from build123d import *

# Parameters (mm, degrees)
SKETCH_1_W          = 40
SKETCH_1_H          = 40
EXTRUDE_1_DEPTH     = 9
SKETCH_2_W          = 5.7
SKETCH_2_H          = 40
EXTRUDE_2_DEPTH     = 40
CUT_EXTRUDE_START   = -40
CUT_EXTRUDE_2_DEPTH = 40
SKETCH_4_R          = 4
CUT_EXTRUDE_3_DEPTH = 67.340033162
SKETCH_5_R          = 8
CUT_EXTRUDE_4_DEPTH = 2
SKETCH_6_R          = 4
CUT_EXTRUDE_5_DEPTH = 49.989794856
SKETCH_7_W          = 8.2
SKETCH_7_H          = 1
EXTRUDE_3_DEPTH     = 2


# Read off the part's stored shape, not the designer's step: 切除-拉伸2
with BuildPart() as part:
    # 草图1 → 凸台-拉伸1 (new body)
    with BuildSketch(Plane.XY):
        Rectangle(SKETCH_1_W, SKETCH_1_H)
    extrude(amount=EXTRUDE_1_DEPTH)

    # 草图2 → 凸台-拉伸2 (add)
    with BuildSketch(Plane.XY.offset(9)):
        with Locations((-17.15, 0)):
            Rectangle(SKETCH_2_W, SKETCH_2_H)
        with Locations((17.15, 0)):
            Rectangle(SKETCH_2_W, SKETCH_2_H)
    extrude(amount=EXTRUDE_2_DEPTH)

    # 切除-拉伸2 outline → 切除-拉伸2 (cut)
    with BuildSketch(Plane.ZY.offset(20).offset(CUT_EXTRUDE_START)):
        with BuildLine():
            Line((49, 20), (29, 20))
            ThreePointArc((29, 20), (43.142135559, 14.142135688), (49, 1.83e-07))
            Line((49, 1.83e-07), (49, 20))
        make_face()
        with BuildLine():
            Line((49, -20), (49, 1.83e-07))
            ThreePointArc((49, 1.83e-07), (43.142135688, -14.142135559), (29, -20))
            Line((29, -20), (49, -20))
        make_face()
    extrude(amount=CUT_EXTRUDE_2_DEPTH, mode=Mode.SUBTRACT)

    # 草图4 → 切除-拉伸3 (cut, through all)
    with BuildSketch(Plane.ZY.offset(20)):
        with Locations((29, 0)):
            Circle(SKETCH_4_R)
    extrude(amount=-CUT_EXTRUDE_3_DEPTH, mode=Mode.SUBTRACT)

    # 草图5 → 切除-拉伸4 (cut)
    with BuildSketch(Plane.ZY.offset(20)):
        with Locations((29, 0)):
            Circle(SKETCH_5_R)
    extrude(amount=-CUT_EXTRUDE_4_DEPTH, mode=Mode.SUBTRACT)

    # 草图6 → 切除-拉伸5 (cut, through all)
    with BuildSketch(Plane.XY.offset(9)):
        Circle(SKETCH_6_R)
    extrude(amount=-CUT_EXTRUDE_5_DEPTH, mode=Mode.SUBTRACT)

    # 草图7 → 凸台-拉伸3 (add)
    with BuildSketch(Plane(origin=(0, 0, 0), x_dir=(-1, 0, 0), z_dir=(0, 0, -1))):
        with Locations((0, 19.5)):
            Rectangle(SKETCH_7_W, SKETCH_7_H)
        with Locations((0, -19.5)):
            Rectangle(SKETCH_7_W, SKETCH_7_H)
    extrude(amount=EXTRUDE_3_DEPTH)


solid = part.part
CAD build for the part. Positions are in the model's coordinates, mm. A direction names the side the tool comes from. Coordinates: 2 decimals unless noted, no trailing zeros. Write each loop counter-clockwise with the first axis right and the second up, starting at its lowest first coordinate (ties: lowest second). Pieces come first, ordered by that corner, then holes. Notation, with made-up numbers: M 41.25,34 L 52.25,34 A21 cw 52.25,67 Z; hole C 8,86.5 d6. An arc over 180 degrees is marked long. Answer as a JSON object with one key per item and string values. Group by question number.
1) Tool access for faces 1 (the face through (-20, 0, 19)), 2 (the face through (0, -19, -1)), 3 (the face through (-19, 0, 21)), 4 (the face through (-14.3, 0, 24)): list every direction of +Z, -Z, +X, -X, +Y, -Y with a clear straight run to the whole face (end or side of a thin tool).
2) Pin check, flat tips, straight feed: pin 1 Ø8 at (x, z) = (7, 39.5) entering from -Y; pin 2 Ø6 at (x, y) = (16, 12) entering from +Z; pin 3 Ø5 at (y, z) = (0.5, 25.5) entering from -X; pin 4 Ø8.5 at (x, y) = (5.5, -1.5) entering from +Z. Stop position of each tip, or through.
3) Saw through at B-B (x = 0). Write the cut outline in (y, z), plus the area to 3 significant figures.
4) Saw through at A-A (z = 5). Write the cut outline in (x, y).
5) Mould opens along Z. For faces 5 (the face through (0, 5, 9)), 6 (the face through (0, 19, -1)), 7 (the face through (-18, -2, 25)) say: +Z half, -Z half, draft (parallel to the pull), parting line (faces both ways), or undercut.
6) Saw through at D-D (x = -17). Write the cut outline in (y, z), plus the area to 3 significant figures.
7) Wall check: line 1 (Y direction, x = 0, z = 2.25); line 2 (X direction, y = 11.5, z = 41); line 3 (Z direction, x = 12.5, y = 2.5). Give the ranges that are in metal, low to high. Write a range as from..to.
8) Saw through at C-C (z = 28). Write the cut outline in (x, y).
Values follow:
{
 "1": {"face 1": "+Z, -Z, -X, +Y, -Y", "face 2": "-Z, +X, -X", "face 3": "-X", "face 4": "+Z, +Y, -Y"},
 "2": {"pin 1": "passes through", "pin 2": "stops at z = 46.86", "pin 3": "stops at x = -18", "pin 4": "stops at z = 9"},
 "3": {"outline": "M -20,-2 L -19,-2 L -19,0 L -4,0 L -4,9 L -20,9 Z; M 4,0 L 19,0 L 19,-2 L 20,-2 L 20,9 L 4,9 Z", "area": "292 mm2"},
 "4": {"outline": "M -20,-20 L 20,-20 L 20,20 L -20,20 Z; hole C 0,0 d8"},
 "5": {"face 5": "+Z half", "face 6": "draft", "face 7": "undercut"},
 "6": {"outline": "M -20,0 L 20,0 L 20,29 A20 ccw -20,29 Z; hole C 0,29 d8", "area": "1,740 mm2"},
 "7": {"line 1": "y = -20..-4, 4..20", "line 2": "x = -20..-14.3, 14.3..20", "line 3": "z = 0..9"},
 "8": {"outline": "M -20,-20 L -14.3,-20 L -14.3,-3.87 L -18,-3.87 L -18,-7.94 L -20,-7.94 Z; M -20,7.94 L -18,7.94 L -18,3.87 L -14.3,3.87 L -14.3,20 L -20,20 Z; M 14.3,-20 L 20,-20 L 20,-3.87 L 14.3,-3.87 Z; M 14.3,3.87 L 20,3.87 L 20,20 L 14.3,20 Z"}
}
